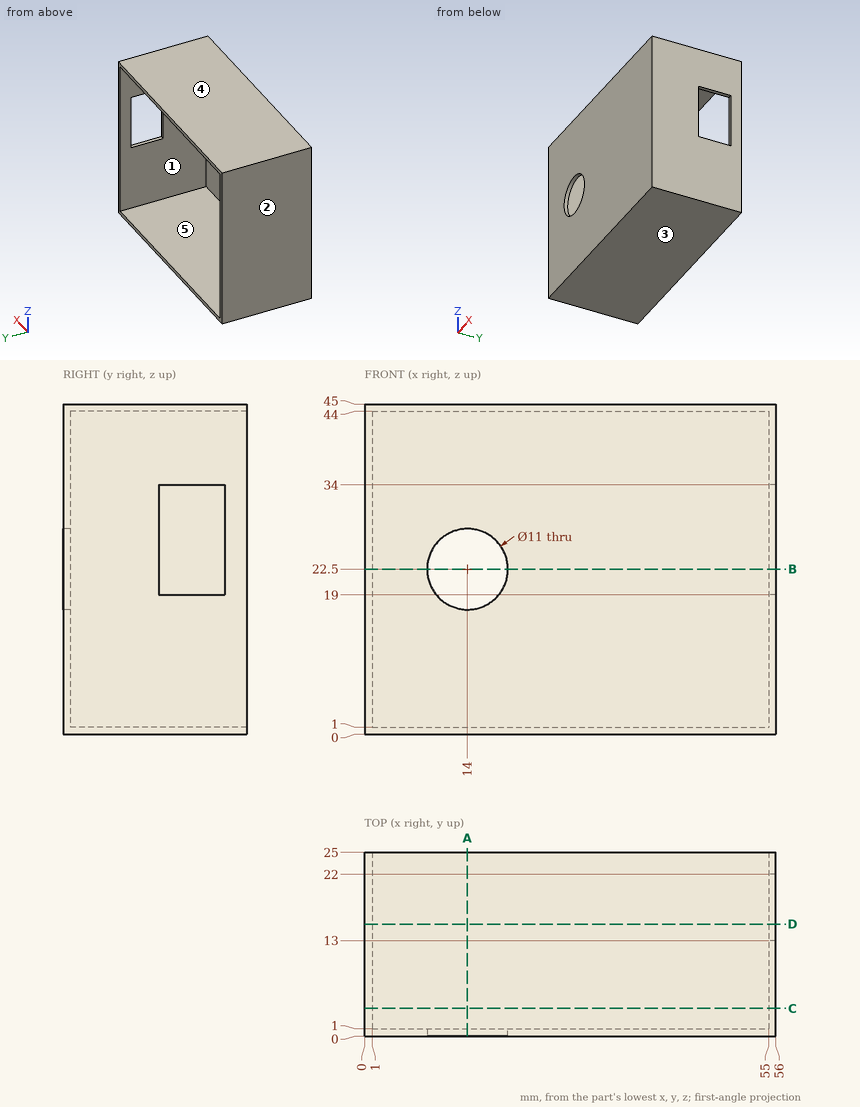
Could you check a few things on this drawing? It's one solid part, dimensions in mm from its lowest x, y, z. A direction names the side the tool comes from. Round coordinates to 2 decimals unless told otherwise and drop trailing zeros. Write each loop counter-clockwise with the first axis right and the second up, starting at its lowest first coordinate (ties: lowest second). Pieces come first, ordered by that corner, then holes. Notation, with made-up numbers: M 77,25.25 L 103,25.25 A10 ccw 103,42.25 Z; hole C -29.75,58.5 d10. An arc over 180 degrees is marked long. Answer as CSV lines item,"result". Start each with the question number.
1. Suppose I cut it at D-D on y = 15.25. Write out the boundary of the cut face in (x, z).
2. Suppose I cut it at B-B on z = 22.5. Write out the boundary of the cut face in (x, y), then the cut area to 3 significant figures.
3. Thinking about a two-plate mould opening in X: for the marked faces 1, 2 and 3, which applies, released by +X, released by -X, zero draft, split by the parting line, or undercut?
4. I'm going to push a flat-ended pin straight in: pin 1 Ø6 at (x, z) = (6.5, 7.5) entering from +Y. Where does the tip first touch, or does it pass through?
5. Suppose I cut it at A-A on x = 14. Write out the boundary of the cut face in (y, z), then the cut area to 3 significant figures.
6. Suppose I cut it at C-C on y = 3.75. Write out the boundary of the cut face in (x, z), then the cut area to 3 significant figures.
7. On a 3-axis mill with a long thin cutter (end or side, diameter ignored), from which of +Z, -Z, +X, -X, +Y, -Y can I reach the whole of each face in a straight line? I mean the marked faces 4 and 5. Say none if no direction works.
8. I need wall thicknesses on probe 1 along X at (y, z) = (14.75, 34.5); probe 2 along Z at (x, y) = (4, 2.5); probe 3 along Z at (x, y) = (14, 0.8). Which ranges of each line are inside material? Lowest first, please.
Check result:
1,outline,"M 0,0 L 56,0 L 56,19 L 55,19 L 55,1 L 1,1 L 1,44 L 55,44 L 55,34 L 56,34 L 56,45 L 0,45 Z"
2,outline,"M 0,0 L 8.5,0 L 8.5,1 L 1,1 L 1,25 L 0,25 Z; M 19.5,0 L 56,0 L 56,13 L 55,13 L 55,1 L 19.5,1 Z; M 55,22 L 56,22 L 56,25 L 55,25 Z"
2,area,"84.0 mm2"
3,face 1,"undercut"
3,face 2,"released by -X"
3,face 3,"zero draft"
4,pin 1,"stops at y = 1"
5,outline,"M 0,0 L 25,0 L 25,1 L 1,1 L 1,17 L 0,17 Z; M 0,28 L 1,28 L 1,44 L 25,44 L 25,45 L 0,45 Z"
5,area,"82.0 mm2"
6,outline,"M 0,0 L 56,0 L 56,45 L 0,45 Z; hole M 1,1 L 55,1 L 55,44 L 1,44 Z"
6,area,"198 mm2"
7,face 4,"+Z, +X, -X, +Y, -Y"
7,face 5,"+Y"
8,probe 1,"x = 0 to 1, 55 to 56"
8,probe 2,"z = 0 to 1, 44 to 45"
8,probe 3,"z = 0 to 17, 28 to 45"
